Source: three-view drawing plus pictorial views. Frame: mm from the lowest corner of the part. Give positions to 0.01 mm unless a question says otherwise; leave off trailing zeros. Order: outer loops, then holes, each group sorted by start corner. A loop starts at its lowest first (then second) coordinate and runs counter-clockwise, first axis right, second up. Notation, with made-up numbers: (43.5, 88) - (63.5, 88) arc R15 ccw to (63.5, 92) - close; hole circle Ø11 at (30, 7.5). An arc over 180 degrees is marked (long way). Answer in a Markdown table with one row per item. Add a question column.
1. Section query A-A on y = 8.5. Return loops of the section in (x, z).
2. Contact query for flat-ended pins moving along their axis: pin 1 (2 mm diameter, centred on x = 117, y = 14.5, fed in from -Z); pin 2 (5.5 mm diameter, centred on x = 82.5, y = 8.5, fed in from -Z). Output: stop coordinate, or through.
3. Section query C-C on z = 6.25. Return loops of the section in (x, y).
4. Section query B-B on x = 82.5. Return loops of the section in (y, z).
5. Section query D-D on x = 38. Return loops of the section in (y, z), and give its area (3 significant figures).
6. Ray query, line 1 (Z direction, x = 109, y = 5.5); line 2 (Y direction, x = 51, z = 8.25); line 3 (Y direction, x = 82.5, z = 1). Return the intervals inside material, ascending. Write a range as [from, to].
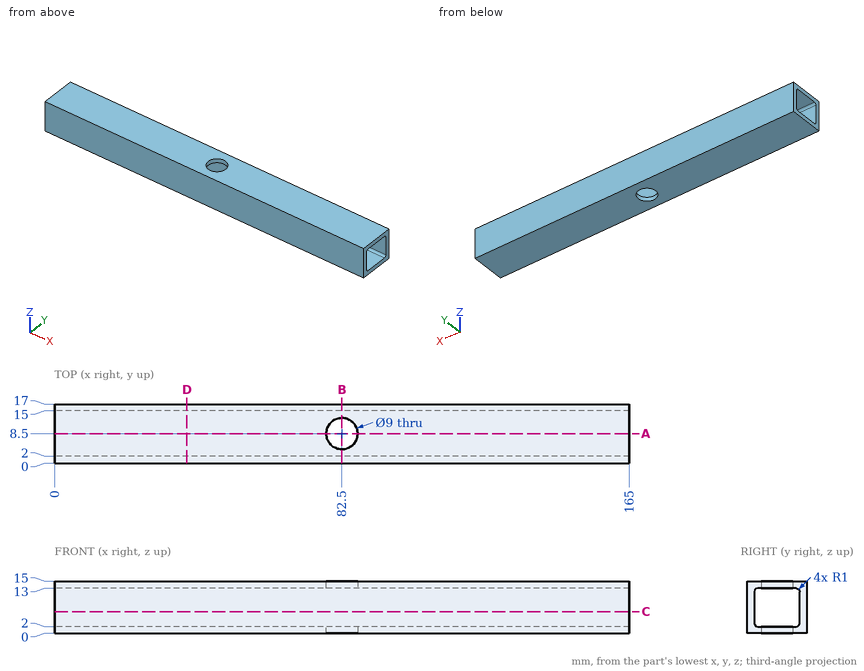
Answer:
| question | item | result |
|---|---|---|
| 1 | outline | (0, 0) - (78, 0) - (78, 2) - (0, 2) - close; (0, 13) - (78, 13) - (78, 15) - (0, 15) - close; (87, 0) - (165, 0) - (165, 2) - (87, 2) - close; (87, 13) - (165, 13) - (165, 15) - (87, 15) - close |
| 2 | pin 1 | stops at z = 0 |
| 2 | pin 2 | passes through |
| 3 | outline | (0, 0) - (165, 0) - (165, 2) - (0, 2) - close; (0, 15) - (165, 15) - (165, 17) - (0, 17) - close |
| 4 | outline | (0, 0) - (4, 0) - (4, 2) - (3, 2) arc R1 cw to (2, 3) - (2, 12) arc R1 cw to (3, 13) - (4, 13) - (4, 15) - (0, 15) - close; (13, 0) - (17, 0) - (17, 15) - (13, 15) - (13, 13) - (14, 13) arc R1 cw to (15, 12) - (15, 3) arc R1 cw to (14, 2) - (13, 2) - close |
| 5 | outline | (0, 0) - (17, 0) - (17, 15) - (0, 15) - close; hole (2, 3) arc R1 ccw to (3, 2) - (14, 2) arc R1 ccw to (15, 3) - (15, 12) arc R1 ccw to (14, 13) - (3, 13) arc R1 ccw to (2, 12) - close |
| 5 | area | 113 mm² |
| 6 | line 1 | z = [0, 2], [13, 15] |
| 6 | line 2 | y = [0, 2], [15, 17] |
| 6 | line 3 | y = [0, 4], [13, 17] |
